```python
from build123d import *
from OCP.BRepFilletAPI import BRepFilletAPI_MakeChamfer

# Parameters (mm, degrees)
SKETCH1_R               = 25
BOSS_EXTRUDE1_DEPTH     = 4
SKETCH2_R               = 19.125
BOSS_EXTRUDE2_DEPTH     = 2.5
SKETCH3_R               = 15.9575
BOSS_EXTRUDE3_DEPTH     = 8
SKETCH4_R               = 2.5
CUT_EXTRUDE1_DEPTH      = 3
SKETCH7_R               = 2.5
CUT_EXTRUDE3_DEPTH      = 11
SKETCH8_R               = 5
CUT_EXTRUDE4_DEPTH      = 4
CHAMFER1_SIZE           = 2.5
FILLET1_R               = 0.5
CUT_EXTRUDE7_DEPTH      = 37.881567212
CUT_EXTRUDE7_DEPTH_BACK = 37.881567212
SKETCH11_R              = 1.65
SKETCH12_R              = 3
CUT_EXTRUDE8_DEPTH      = 5
CUT_EXTRUDE11_START     = -5
SKETCH15_R              = 5
CUT_EXTRUDE11_DEPTH     = 5
CHAMFER2_SIZE           = 1.5
FILLET2_R               = 2
CHAMFER3_SIZE           = 1.5
CHAMFER3_SIZE2          = 0.264490471
CHAMFER4_SIZE           = 0.75
CHAMFER5_SIZE           = 0.75
SKETCH16_R              = 0.75
CUT_EXTRUDE12_DEPTH     = 38.027017163
CHAMFER6_SIZE           = 0.4
DRAFT1_ANGLE            = 1.75
DRAFT2_ANGLE            = 1


with BuildPart() as part:
    # Sketch1 → Boss-Extrude1 (new body)
    with BuildSketch(Plane.XY):
        Circle(SKETCH1_R)
    extrude(amount=BOSS_EXTRUDE1_DEPTH)

    # Sketch2 → Boss-Extrude2 (add)
    with BuildSketch(Plane.XY.offset(4)):
        Circle(SKETCH2_R)
    extrude(amount=BOSS_EXTRUDE2_DEPTH)

    # Sketch3 → Boss-Extrude3 (add)
    with BuildSketch(Plane.XY.offset(6.5)):
        Circle(SKETCH3_R)
    extrude(amount=BOSS_EXTRUDE3_DEPTH)

    # Sketch4 → Cut-Extrude1 (cut)
    with BuildSketch(Plane(origin=(0, 0, 0), x_dir=(-1, 0, 0), z_dir=(0, 0, -1))):
        with Locations((0, 16.93333)):
            Circle(SKETCH4_R)
        with Locations((16.93333, 0)):
            Circle(SKETCH4_R)
        with Locations((0, -16.93333)):
            Circle(SKETCH4_R)
        with Locations((-16.93333, 0)):
            Circle(SKETCH4_R)
    extrude(amount=-CUT_EXTRUDE1_DEPTH, mode=Mode.SUBTRACT)

    # Sketch7 → Cut-Extrude3 (cut)
    with BuildSketch(Plane.XY.offset(14.5)):
        with Locations((0, 11)):
            Circle(SKETCH7_R)
        with Locations((9.526279442, 5.5)):
            Circle(SKETCH7_R)
        with Locations((9.526279442, -5.5)):
            Circle(SKETCH7_R)
        with Locations((0, -11)):
            Circle(SKETCH7_R)
        with Locations((-9.526279442, -5.5)):
            Circle(SKETCH7_R)
        with Locations((-9.526279442, 5.5)):
            Circle(SKETCH7_R)
    extrude(amount=-CUT_EXTRUDE3_DEPTH, mode=Mode.SUBTRACT)

    # Sketch8 → Cut-Extrude4 (cut)
    with BuildSketch(Plane(origin=(0, 0, 0), x_dir=(-1, 0, 0), z_dir=(0, 0, -1))):
        Circle(SKETCH8_R)
    extrude(amount=-CUT_EXTRUDE4_DEPTH, mode=Mode.SUBTRACT)

    # Chamfer1
    chamfer1_edges = [part.edges().sort_by_distance(p)[0] for p in [
        (-25, 0, 0),
    ]]
    chamfer(chamfer1_edges, length=CHAMFER1_SIZE)

    # Fillet1
    fillet1_edges = [part.edges().sort_by_distance(p)[0] for p in [
        (-15.9575, 0, 14.5),
    ]]
    fillet(fillet1_edges, radius=FILLET1_R)

    # Sketch11 → Cut-Extrude7 (cut, two sides: drawn at the far end of the back side and taken through both)
    with BuildSketch(Plane.XY.offset(4).offset(-CUT_EXTRUDE7_DEPTH_BACK)):
        with Locations((-13.435028843, 13.435028843)):
            Circle(SKETCH11_R)
        with Locations((13.435028843, 13.435028843)):
            Circle(SKETCH11_R)
        with Locations((13.435028843, -13.435028843)):
            Circle(SKETCH11_R)
        with Locations((-13.435028843, -13.435028843)):
            Circle(SKETCH11_R)
    extrude(amount=CUT_EXTRUDE7_DEPTH + CUT_EXTRUDE7_DEPTH_BACK, mode=Mode.SUBTRACT)

    # Sketch12 → Cut-Extrude8 (cut)
    with BuildSketch(Plane.XY.offset(6.5)):
        with Locations((-13.435028843, 13.435028843)):
            Circle(SKETCH12_R)
        with Locations((13.435028843, 13.435028843)):
            Circle(SKETCH12_R)
        with Locations((13.435028843, -13.435028843)):
            Circle(SKETCH12_R)
        with Locations((-13.435028843, -13.435028843)):
            Circle(SKETCH12_R)
    extrude(amount=-CUT_EXTRUDE8_DEPTH, mode=Mode.SUBTRACT)

    # Sketch15 → Cut-Extrude11 (cut)
    with BuildSketch(Plane.XY.offset(14.5).offset(CUT_EXTRUDE11_START)):
        with Locations(Location((0, 0, 0), (0, 0, 180))):
            Circle(SKETCH15_R)
    extrude(amount=CUT_EXTRUDE11_DEPTH, mode=Mode.SUBTRACT)

    # Chamfer2
    # the kernel refuses this chamfer: 1.5 mm, written as the material it adds along each edge
    with BuildSketch(Plane(origin=(13.435028843, -13.435028843, 1.5), x_dir=(1, 0, 0), z_dir=(0, -1, 0))) as chamfer2_piece_1_section:
        Polygon((3, CHAMFER2_SIZE), (3 - CHAMFER2_SIZE, 0), (3, 0), align=None)
    chamfer2_piece_1 = revolve(axis=Axis((13.435028843, -13.435028843, 1.5), (0, 0, 1)), mode=Mode.PRIVATE)
    chamfer2_piece_1 = chamfer2_piece_1 - Plane(origin=(13.435028843, -13.435028843, 2.327258636), x_dir=(1, 0, 0), z_dir=(0, 0, 1)) * Cylinder(1.65, 13, mode=Mode.PRIVATE)
    add(chamfer2_piece_1)
    with BuildSketch(Plane(origin=(-13.435028843, -13.435028843, 1.5), x_dir=(1, 0, 0), z_dir=(0, -1, 0))) as chamfer2_piece_2_section:
        Polygon((3, CHAMFER2_SIZE), (3 - CHAMFER2_SIZE, 0), (3, 0), align=None)
    chamfer2_piece_2 = revolve(axis=Axis((-13.435028843, -13.435028843, 1.5), (0, 0, 1)), mode=Mode.PRIVATE)
    chamfer2_piece_2 = chamfer2_piece_2 - Plane(origin=(-13.435028843, -13.435028843, 2.327258636), x_dir=(1, 0, 0), z_dir=(0, 0, 1)) * Cylinder(1.65, 12, mode=Mode.PRIVATE)
    add(chamfer2_piece_2)
    with BuildSketch(Plane(origin=(13.435028843, 13.435028843, 1.5), x_dir=(1, 0, 0), z_dir=(0, -1, 0))) as chamfer2_piece_3_section:
        Polygon((3, CHAMFER2_SIZE), (3 - CHAMFER2_SIZE, 0), (3, 0), align=None)
    chamfer2_piece_3 = revolve(axis=Axis((13.435028843, 13.435028843, 1.5), (0, 0, 1)), mode=Mode.PRIVATE)
    chamfer2_piece_3 = chamfer2_piece_3 - Plane(origin=(13.435028843, 13.435028843, 2.327258636), x_dir=(1, 0, 0), z_dir=(0, 0, 1)) * Cylinder(1.65, 13, mode=Mode.PRIVATE)
    add(chamfer2_piece_3)
    with BuildSketch(Plane(origin=(-13.435028843, 13.435028843, 1.5), x_dir=(1, 0, 0), z_dir=(0, -1, 0))) as chamfer2_piece_4_section:
        Polygon((3, CHAMFER2_SIZE), (3 - CHAMFER2_SIZE, 0), (3, 0), align=None)
    chamfer2_piece_4 = revolve(axis=Axis((-13.435028843, 13.435028843, 1.5), (0, 0, 1)), mode=Mode.PRIVATE)
    chamfer2_piece_4 = chamfer2_piece_4 - Plane(origin=(-13.435028843, 13.435028843, 2.327258636), x_dir=(1, 0, 0), z_dir=(0, 0, 1)) * Cylinder(1.65, 13, mode=Mode.PRIVATE)
    add(chamfer2_piece_4)

    # Fillet2
    fillet2_edges = [part.edges().sort_by_distance(p)[0] for p in [
        (5, 0, 4),
    ]]
    fillet(fillet2_edges, radius=FILLET2_R)

    # Chamfer3: one chamfer whose edges measure the first distance from different faces: ONE call of the kernel's chamfer builder (chamfer() names one face for all edges)
    chamfer3_edges_1 = [part.edges().sort_by_distance(p)[0] for p in [
        (0, -19.125, 6.5),
    ]]
    chamfer3_side_1 = [part.faces().sort_by_distance(p)[0] for p in [
        (0, -19.125, 5.25),
    ]]
    chamfer3_edges_2 = [part.edges().sort_by_distance(p)[0] for p in [
        (19.125, 0, 6.5),
    ]]
    chamfer3_side_2 = [part.faces().sort_by_distance(p)[0] for p in [
        (19.125, 0, 5.25),
    ]]
    chamfer3_edges_3 = [part.edges().sort_by_distance(p)[0] for p in [
        (0, 19.125, 6.5),
    ]]
    chamfer3_side_3 = [part.faces().sort_by_distance(p)[0] for p in [
        (0, 19.125, 5.25),
    ]]
    chamfer3_edges_4 = [part.edges().sort_by_distance(p)[0] for p in [
        (-19.125, 0, 6.5),
    ]]
    chamfer3_side_4 = [part.faces().sort_by_distance(p)[0] for p in [
        (-19.125, 0, 5.25),
    ]]
    chamfer3 = BRepFilletAPI_MakeChamfer(part.part.solid().wrapped)
    for e in chamfer3_edges_1:
        chamfer3.Add(CHAMFER3_SIZE, CHAMFER3_SIZE2, e.wrapped, chamfer3_side_1[0].wrapped)  # the first distance lies on this face
    for e in chamfer3_edges_2:
        chamfer3.Add(CHAMFER3_SIZE, CHAMFER3_SIZE2, e.wrapped, chamfer3_side_2[0].wrapped)  # the first distance lies on this face
    for e in chamfer3_edges_3:
        chamfer3.Add(CHAMFER3_SIZE, CHAMFER3_SIZE2, e.wrapped, chamfer3_side_3[0].wrapped)  # the first distance lies on this face
    for e in chamfer3_edges_4:
        chamfer3.Add(CHAMFER3_SIZE, CHAMFER3_SIZE2, e.wrapped, chamfer3_side_4[0].wrapped)  # the first distance lies on this face
    add(Compound.cast(chamfer3.Shape()), mode=Mode.REPLACE)

    # Chamfer4
    chamfer4_edges = [part.edges().sort_by_distance(p)[0] for p in [
        (5, 0, 9.5),
    ]]
    chamfer(chamfer4_edges, length=CHAMFER4_SIZE)

    # Chamfer5
    chamfer5_edges = [part.edges().sort_by_distance(p)[0] for p in [
        (5, 0, 14.5),
    ]]
    chamfer(chamfer5_edges, length=CHAMFER5_SIZE)

    # Sketch16 → Cut-Extrude12 (cut, through all)
    with BuildSketch(Plane.XY.offset(3.5)):
        with Locations((-9.526279442, -5.5)):
            Circle(SKETCH16_R)
        with Locations((-9.526279442, 5.5)):
            Circle(SKETCH16_R)
        with Locations((0, 11)):
            Circle(SKETCH16_R)
        with Locations((9.526279442, 5.5)):
            Circle(SKETCH16_R)
        with Locations((9.526279442, -5.5)):
            Circle(SKETCH16_R)
        with Locations((0, -11)):
            Circle(SKETCH16_R)
    extrude(amount=-CUT_EXTRUDE12_DEPTH, mode=Mode.SUBTRACT)

    # Chamfer6
    chamfer6_edges = [part.edges().sort_by_distance(p)[0] for p in [
        (2.5, 16.93333, 0),
        (-14.43333, 0, 0),
        (2.5, -16.93333, 0),
        (19.43333, 0, 0),
    ]]
    chamfer(chamfer6_edges, length=CHAMFER6_SIZE)

    # Draft1
    draft1_faces = [part.faces().sort_by_distance(p)[0] for p in [
        (7.026279442, 5.5, 9),
        (-2.5, 11, 9),
        (-12.026279442, 5.5, 9),
        (-12.026279442, -5.5, 9),
        (-2.5, -11, 9),
        (7.026279442, -5.5, 9),
    ]]
    draft(draft1_faces, Plane(origin=(9.526279442, -5.5, 3.5), x_dir=(1, 0, 0), z_dir=(0, 0, 1)), DRAFT1_ANGLE)

    # Draft2
    draft2_faces = [part.faces().sort_by_distance(p)[0] for p in [
        (2.5, -16.93333, 1.7),
        (-14.43333, 0, 1.7),
        (19.43333, 0, 1.7),
        (2.5, 16.93333, 1.7),
    ]]
    draft(draft2_faces, Plane(origin=(0, 16.93333, 3), x_dir=(-1, 0, 0), z_dir=(0, 0, -1)), DRAFT2_ANGLE)


solid = part.part
```
Source: CAD feature listing. Evaluate the final solid. Frame: model axes, mm. A direction names the side the tool comes from. Coordinates: 2 decimals unless noted, no trailing zeros. Loops run counter-clockwise (first coordinate to the right, second up) from the corner with the lowest first, then second, coordinate; pieces in that order, holes last. Notation, with made-up numbers: M -6,-25.5 L 47,-25.5 A6 ccw 47,-16.5 Z; hole C 36,48.25 d5. An arc over 180 degrees is marked long. Use a Markdown table: item, result. Add a question column.
Q1. Access query for faces 4 (the cylindrical face through (-13.65, -11.8, 0.81)), 5 (the flat face through (0, -17, 3)), 6 (the cylindrical face through (-10.574, -12.534, 4.386)). Directions: +Z, -Z, +X, -X, +Y, -Y. A direction counts if a zero-diameter tool reaches every point of the face in a straight line with its end or side. Return the directions, or none.
Q2. Material intervals for L1, parallel to Y at x = -8, z = 10; L2, parallel to X at y = -6, z = 7.5; L3, parallel to Y at x = 9, z = 5.75, sorted ascending.
Q3. Section query A-A, the plane z = 8.5. Return loops of the section in (x, y) (1 decimal).
Q4. Section query C-C, the plane x = 0. State how many separate pieces and enclosed holes the cut face has, and give its area (3 significant figures).
Q5. First-contact query: pin 1 (0.9 mm diameter, centred on x = -9.53, y = 5.5, fed in from -Z); pin 2 (8 mm diameter, centred on x = 0, y = 0, fed in from -Z); pin 3 (2 mm diameter, centred on x = -5.5, y = 18, fed in from +Z); pin 4 (5 mm diameter, centred on x = 0.5, y = 1, fed in from -Z). Flat tips, straight axial feed; report the tip coordinate or a pass-through.
Q6. Section query B-B, the plane z = 13. Return loops of the section in (x, y) (1 decimal), and give its area (3 significant figures).
Q7. Draft query along X for faces 1 (the conical face through (0.17, 18.96, 5.93)), 2 (the flat face through (11, -17, 4)), 3 (the flat face through (-10, -7, 3.5)). Return one class per face: pulls with the +X half, pulls with the -X half, needs draft (parallel to the pull), parting line crosses it, or undercut.
Result:
| question | item | result |
|---|---|---|
| 1 | face 4 | +Z, -Z |
| 1 | face 5 | -Z |
| 1 | face 6 | +Z |
| 2 | L1 | y = -13.81 to -7.73, -3.27 to 3.27, 7.73 to 13.81 |
| 2 | L2 | x = -14.79 to -12.1, -6.95 to 6.95, 12.1 to 14.79 |
| 2 | L3 | y = -16.72 to -8.01, -2.99 to 2.99, 8.01 to 16.72 |
| 3 | outline | C 0,0 d31.9; hole C -9.5,-5.5 d5.3; hole C -9.5,5.5 d5.3; hole C 0,-11 d5.3; hole C 0,11 d5.3; hole C 9.5,-5.5 d5.3; hole C 9.5,5.5 d5.3 |
| 4 | separate pieces | 3 |
| 4 | enclosed holes | 0 |
| 4 | area | 297 mm2 |
| 5 | pin 1 | passes through |
| 5 | pin 2 | stops at z = 3.73 |
| 5 | pin 3 | stops at z = 6.5 |
| 5 | pin 4 | stops at z = 3.9 |
| 6 | outline | C 0,0 d31.9; hole C -9.5,-5.5 d5.6; hole C -9.5,5.5 d5.6; hole C 0,0 d10; hole C 0,-11 d5.6; hole C 0,11 d5.6; hole C 9.5,-5.5 d5.6; hole C 9.5,5.5 d5.6 |
| 6 | area | 575 mm2 |
| 7 | face 1 | parting line crosses it |
| 7 | face 2 | needs draft |
| 7 | face 3 | undercut |
